Input: dimensioned drawing with shaded views. Units: mm. Origin: part minimum x, y, z. A direction names the side the tool comes from. Round coordinates to 2 decimals unless told otherwise and drop trailing zeros. Loops run counter-clockwise (first coordinate to the right, second up) from the corner with the lowest first, then second, coordinate; pieces in that order, holes last. Notation, with made-up numbers: (22.25, -18.5) - (50.25, -18.5) arc R24 ccw to (50.25, -6.5) - close; hole circle Ø11 at (86, 8.25). An arc over 180 degrees is marked (long way). Answer as CSV lines item,"result".
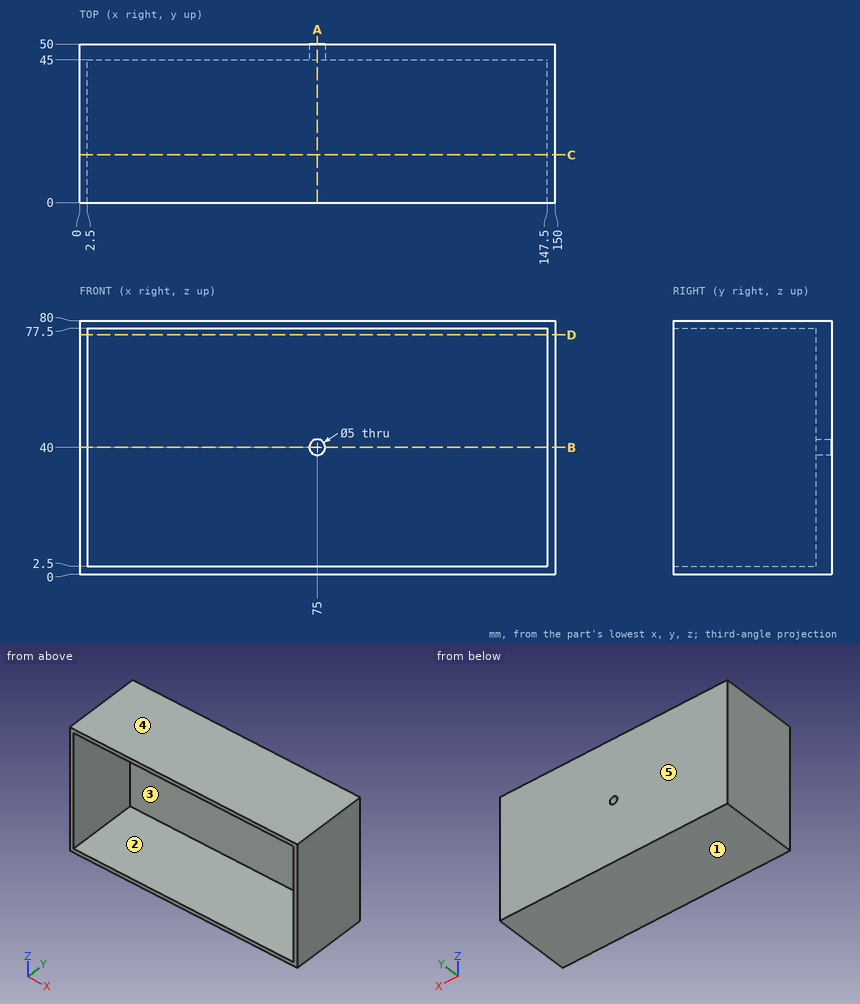
(1) Section C-C (y = 15). Output: boundary loops of the cut face in (x, z), and give its area (4 significant figures).
Findings below:
outline,"(0, 0) - (150, 0) - (150, 80) - (0, 80) - close; hole (2.5, 2.5) - (147.5, 2.5) - (147.5, 77.5) - (2.5, 77.5) - close"
area,"1,125 mm2"
(2) Material intervals for line 1 along X through (y, z) = (26.5, 13); line 2 along Z through (x, y) = (75, 47); line 3 along Z through (x, y) = (21, 20.5), sorted ascending.
Findings below:
line 1,"0 to 2.5, 147.5 to 150"
line 2,"0 to 37.5, 42.5 to 80"
line 3,"0 to 2.5, 77.5 to 80"
(3) Draft query along Z for the marked faces 3, 4 and 5. Return one class per face: pulls with the +Z half, pulls with the -Z half, needs draft (parallel to the pull), parting line crosses it, or undercut.
Findings below:
face 3,"undercut"
face 4,"pulls with the +Z half"
face 5,"needs draft"
(4) Section D-D (z = 75.5). Output: boundary loops of the cut face in (x, y), and give its area (3 significant figures).
Findings below:
outline,"(0, 0) - (2.5, 0) - (2.5, 45) - (147.5, 45) - (147.5, 0) - (150, 0) - (150, 50) - (0, 50) - close"
area,"975 mm2"
(5) Section A-A (x = 75). Output: boundary loops of the cut face in (y, z).
Findings below:
outline,"(0, 0) - (50, 0) - (50, 37.5) - (45, 37.5) - (45, 2.5) - (0, 2.5) - close; (0, 77.5) - (45, 77.5) - (45, 42.5) - (50, 42.5) - (50, 80) - (0, 80) - close"
(6) Section B-B (z = 40). Output: boundary loops of the cut face in (x, y), and give its area (3 significant figures).
Findings below:
outline,"(0, 0) - (2.5, 0) - (2.5, 45) - (72.5, 45) - (72.5, 50) - (0, 50) - close; (77.5, 45) - (147.5, 45) - (147.5, 0) - (150, 0) - (150, 50) - (77.5, 50) - close"
area,"950 mm2"
(7) Access query for the marked faces 1 and 2. Directions: +Z, -Z, +X, -X, +Y, -Y. A direction counts if a zero-diameter tool reaches every point of the face in a straight line with its end or side. Return the directions, or none.
Findings below:
face 1,"-Z, +X, -X, +Y, -Y"
face 2,"-Y"
(8) Pin query (flat end, axial travel): P1, Ø22.5, axis at x = 105.5, z = 26.5, coming from the -Y side. Return the tip coordinate at first contact, or that it passes through.
Findings below:
P1,"y = 45"
